For this review, use the dimensioned drawing (mm, ordinates from the lowest corner) and the shaded views. Give positions to 0.01 mm unless a question says otherwise; leave off trailing zeros. Order: outer loops, then holes, each group sorted by start corner. A loop starts at its lowest first (then second) coordinate and runs counter-clockwise, first axis right, second up. Notation, with made-up numbers: M -34.5,63.5 L -25.5,63.5 A13 ccw -25.5,75.5 Z; hole C 59.25,-24.5 d10. An arc over 180 degrees is marked long. One line per question, with ' | ' between items. Start each with the question number.
1. The part is to be moulded in two halves that separate along Z. For the marked faces 1 and 2, say which applies: +Z half, -Z half, draft (parallel to the pull), parting line (faces both ways), or undercut.
2. We need section D-D on y = 9. Write out the cut boundary in (x, z), then the cut area to 3 significant figures.
3. We need section C-C on z = 2.65. Write out the cut boundary in (x, y), then the cut area to 3 significant figures.
4. Wall thickness on L1, parallel to X at y = 19, z = 3.8; L2, parallel to Y at x = 95.5, z = 2.1; L3, parallel to X at y = 16, z = 3.25: over which ranges is each line inside the solid? List them lowest first.
5. Insertion check: P1, Ø4, axis at x = 61, y = 31, coming from the -Z side. The pin has a flat end and moves straight along its axis. Give the tip position at first contact, or say it passes through.
6. We need section B-B on x = 134.5. Write out the cut boundary in (y, z), then the cut area to 3 significant figures.
7. We need section A-A on y = 19.5. Write out the cut boundary in (x, z).
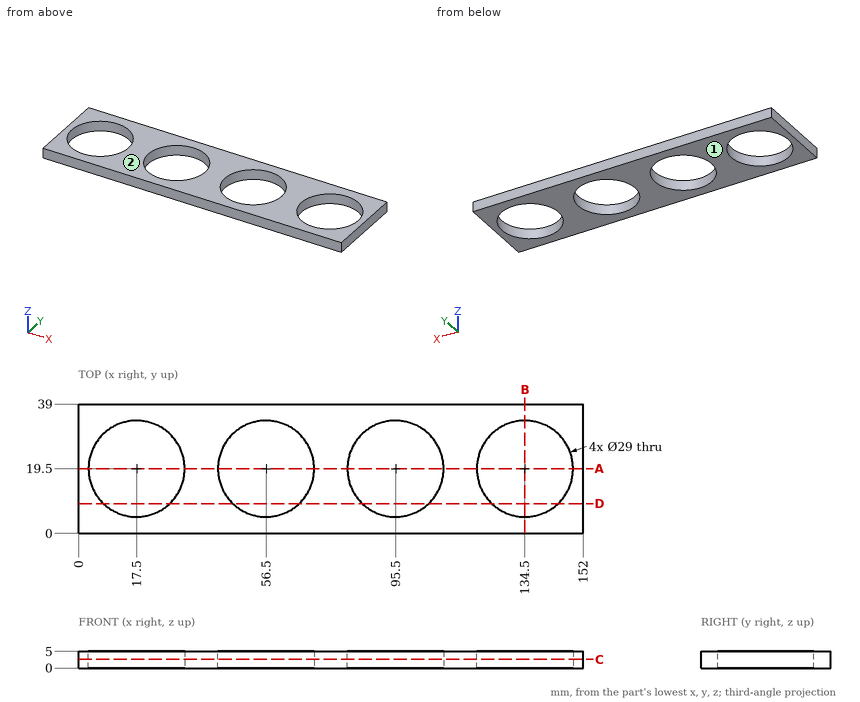
Entries:
1) face 1: -Z half | face 2: +Z half
2) outline: M 0,0 L 7.5,0 L 7.5,5 L 0,5 Z; M 27.5,0 L 46.5,0 L 46.5,5 L 27.5,5 Z; M 66.5,0 L 85.5,0 L 85.5,5 L 66.5,5 Z; M 105.5,0 L 124.5,0 L 124.5,5 L 105.5,5 Z; M 144.5,0 L 152,0 L 152,5 L 144.5,5 Z | area: 360 mm^2
3) outline: M 0,0 L 152,0 L 152,39 L 0,39 Z; hole C 17.5,19.5 d29; hole C 56.5,19.5 d29; hole C 95.5,19.5 d29; hole C 134.5,19.5 d29 | area: 3,290 mm^2
4) L1: x = 0 to 3.01, 31.99 to 42.01, 70.99 to 81.01, 109.99 to 120.01, 148.99 to 152 | L2: y = 0 to 5, 34 to 39 | L3: x = 0 to 3.43, 31.57 to 42.43, 70.57 to 81.43, 109.57 to 120.43, 148.57 to 152
5) P1: passes through
6) outline: M 0,0 L 5,0 L 5,5 L 0,5 Z; M 34,0 L 39,0 L 39,5 L 34,5 Z | area: 50.0 mm^2
7) outline: M 0,0 L 3,0 L 3,5 L 0,5 Z; M 32,0 L 42,0 L 42,5 L 32,5 Z; M 71,0 L 81,0 L 81,5 L 71,5 Z; M 110,0 L 120,0 L 120,5 L 110,5 Z; M 149,0 L 152,0 L 152,5 L 149,5 Z
